```python
from build123d import *

# Parameters (mm, degrees)
BOSS_EXTRUDE1_DEPTH = 6
SKETCH2_R           = 2
CUT_EXTRUDE1_DEPTH  = 8


with BuildPart() as part:
    # Sketch1 → Boss-Extrude1 (new body)
    with BuildSketch(Plane.XY):
        with BuildLine():
            Line((-8, 3.1), (8, 3.1))
            ThreePointArc((8, 3.1), (8.925, 2.479967104), (8.702939142, 1.38875))
            Line((8.702939142, 1.38875), (4.214189142, -3.1))
            Line((4.214189142, -3.1), (-4.214189142, -3.1))
            Line((-4.214189142, -3.1), (-8.702939142, 1.38875))
            ThreePointArc((-8.702939142, 1.38875), (-8.925, 2.479967104), (-8, 3.1))
        make_face()
    extrude(amount=BOSS_EXTRUDE1_DEPTH)

    # Sketch2 → Cut-Extrude1 (cut)
    with BuildSketch(Plane(origin=(0, 3.1, 0), x_dir=(1, 0, 0), z_dir=(0, 1, 0))):
        with Locations((0, -3)):
            Circle(SKETCH2_R)
    extrude(amount=-CUT_EXTRUDE1_DEPTH, mode=Mode.SUBTRACT)


solid = part.part
```
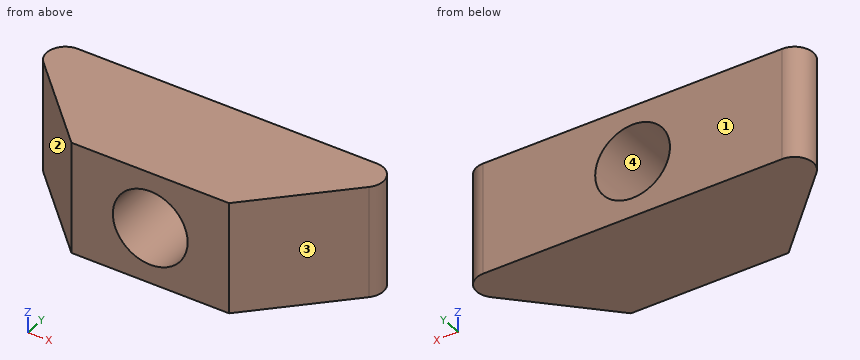
Build history of the part. All positions in model axes, mm. Face numbers are marked on the shaded views. Give positions to 0.01 mm unless a question says otherwise; leave off trailing zeros. Loops run counter-clockwise (first coordinate to the right, second up) from the corner with the lowest first, then second, coordinate; pieces in that order, holes last.
1) Band-saw the part on D-D on z = 4.1. List the corners of the cut face in (x, y).
Values follow:
outline: (-8.7, 1.39) - (-4.21, -3.1) - (-1.67, -3.1) - (-1.67, 3.1) - (-8, 3.1) arc R1 ccw to start; (1.67, -3.1) - (4.21, -3.1) - (8.7, 1.39) arc R1 ccw to (8, 3.1) - (1.67, 3.1) - close
2) Band-saw the part on C-C on y = -1.25. List the corners of the cut face in (x, z).
Values follow:
outline: (-6.06, 0) - (6.06, 0) - (6.06, 6) - (-6.06, 6) - close; hole circle Ø4 at (0, 3)
3) Band-saw the part on A-A on z = 3. List the corners of the cut face in (x, y), then the cut area to 3 significant figures.
Values follow:
outline: (-8.7, 1.39) - (-4.21, -3.1) - (-2, -3.1) - (-2, 3.1) - (-8, 3.1) arc R1 ccw to start; (2, -3.1) - (4.21, -3.1) - (8.7, 1.39) arc R1 ccw to (8, 3.1) - (2, 3.1) - close
area: 63.4 mm2
4) Probe line 1 along Z through (x, y) = (0, 0.75); line 2 along X through (y, z) = (1.25, 3); line 3 along X through (y, z) = (-1.25, 1.9). List the from-to ranges inside material, lowest first.
Values follow:
line 1: z = 0 to 1, 5 to 6
line 2: x = -8.56 to -2, 2 to 8.56
line 3: x = -6.06 to -1.67, 1.67 to 6.06
5) Band-saw the part on B-B on x = 0. List the corners of the cut face in (y, z).
Values follow:
outline: (-3.1, 0) - (3.1, 0) - (3.1, 1) - (-3.1, 1) - close; (-3.1, 5) - (3.1, 5) - (3.1, 6) - (-3.1, 6) - close
6) Two-plate mould, pull along X, no slides. Class the marked faces 1, 2, 3 and 4: released by +X, released by -X, zero draft, split by the parting line, or undercut.
Values follow:
face 1: zero draft
face 2: released by -X
face 3: released by +X
face 4: undercut
